Could you check a few things on this model? Use its own coordinates, in mm. A direction names the side the tool comes from. Round coordinates to 2 decimals unless told otherwise and drop trailing zeros. Order: outer loops, then holes, each group sorted by start corner. A loop starts at its lowest first (then second) coordinate and runs counter-clockwise, first axis right, second up. Notation, with made-up numbers: (34.25, -36.75) -> (41.25, -36.75) arc R24 ccw to (41.25, 1.25) -> close; hole circle Ø9 at (42, 8.25). An arc over 180 degrees is marked (long way). One line per question, with ' | ' between items.
```python
from build123d import *
from build123d.topology import SkipClean

# Parameters (mm, degrees)
SKETCH2_R           = 5.25
BOSS_EXTRUDE1_DEPTH = 14
CUT_EXTRUDE1_DEPTH  = 1
CUT_EXTRUDE2_DEPTH  = 1
BOSS_EXTRUDE2_DEPTH = 9
BOSS_EXTRUDE3_DEPTH = 9.5
FILLET1_R           = 1


with BuildPart() as part:
    # Sketch2 → Boss-Extrude1 (new body)
    with BuildSketch(Plane(origin=(0, 0, 0), x_dir=(0, 0, -1), z_dir=(1, 0, 0))):
        with BuildLine():
            ThreePointArc((0, 0), (9, 9), (0, 18))
            Line((0, 18), (-4.055355956, 18))
            Line((-4.055355956, 18), (-14.1, 8.3))
            Line((-14.1, 8.3), (-22.975773924, 5.754912782))
            ThreePointArc((-22.975773924, 5.754912782), (-23.743647767, 6.106105344), (-24.576075178, 6.24763647))
            Line((-24.576075178, 6.24763647), (-45.007968978, 23.392031022))
            Line((-45.007968978, 23.392031022), (-47.2, 21.2))
            Line((-47.2, 21.2), (-27.661634154, 1.661634154))
            ThreePointArc((-27.661634154, 1.661634154), (-25.892761453, -0.023213541), (-23.45, 0))
            Line((-23.45, 0), (0, 0))
        make_face()
        with Locations((0, 9)):
            Circle(SKETCH2_R, mode=Mode.SUBTRACT)
    extrude(amount=-BOSS_EXTRUDE1_DEPTH)

    # Sketch2_5 → Cut-Extrude1 (cut)
    with BuildSketch(Plane(origin=(0, 0, 0), x_dir=(0, 0, -1), z_dir=(1, 0, 0))):
        with BuildLine():
            Line((-29.259155366, 3.259155366), (-27.661634154, 1.661634154))
            ThreePointArc((-27.661634154, 1.661634154), (-27.396479719, 4.814248364), (-24.576075178, 6.24763647))
            Line((-24.576075178, 6.24763647), (-25.89413767, 7.35362222))
            ThreePointArc((-25.89413767, 7.35362222), (-25.722467199, 6.887608312), (-26.037233654, 6.503470587))
            ThreePointArc((-26.037233654, 6.503470587), (-27.626659815, 5.344602808), (-28.410825273, 3.540625374))
            ThreePointArc((-28.410825273, 3.540625374), (-28.748146118, 3.138148273), (-29.259155366, 3.259155366))
        make_face()
    extrude(amount=-CUT_EXTRUDE1_DEPTH, mode=Mode.SUBTRACT)

    # Sketch2_6 → Cut-Extrude2 (cut)
    with SkipClean():  # the faces are left unmerged after this step: merging them gives an invalid solid
        with BuildSketch(Plane(origin=(0, 0, 0), x_dir=(0, 0, -1), z_dir=(1, 0, 0))):
            with BuildLine():
                Line((-23.45, 0), (-21.263068229, 0))
                ThreePointArc((-21.263068229, 0), (-21.708634623, 0.273128697), (-21.667413143, 0.794117647))
                ThreePointArc((-21.667413143, 0.794117647), (-20.951415597, 3.103028999), (-21.793156226, 5.369126268))
                ThreePointArc((-21.793156226, 5.369126268), (-21.882671913, 5.8346109), (-21.543395734, 6.165640619))
                Line((-21.543395734, 6.165640619), (-22.975773924, 5.754912782))
                ThreePointArc((-22.975773924, 5.754912782), (-21.856917628, 4.574605546), (-21.45, 3))
                ThreePointArc((-21.45, 3), (-21.995836543, 1.197224362), (-23.45, 0))
            make_face()
        extrude(amount=-CUT_EXTRUDE2_DEPTH, mode=Mode.SUBTRACT)

    # Sketch3 → Boss-Extrude2 (add)
    with SkipClean():  # the faces are left unmerged after this step: merging them gives an invalid solid
        with BuildSketch(Plane.ZY.offset(14)):
            with BuildLine():
                ThreePointArc((23.45, 0), (21.46097847, 2.733092659), (22.975773924, 5.754912782))
                Line((22.975773924, 5.754912782), (14.1, 8.3))
                Line((14.1, 8.3), (11.259590113, 9.114474429))
                ThreePointArc((11.259590113, 9.114474429), (10.41329932, 8.974403731), (9.986911251, 8.230077781))
                ThreePointArc((9.986911251, 8.230077781), (9.041706899, 4.689696888), (6.886416056, 1.726180477))
                ThreePointArc((6.886416056, 1.726180477), (6.644893676, 0.629986809), (7.573920177, 0))
                Line((7.573920177, 0), (23.45, 0))
            make_face()
            with BuildLine():
                ThreePointArc((27.95, 3), (26.953857175, 5.341501193), (24.576075178, 6.24763647))
                ThreePointArc((24.576075178, 6.24763647), (23.743647767, 6.106105344), (22.975773924, 5.754912782))
                ThreePointArc((22.975773924, 5.754912782), (21.46097847, 2.733092659), (23.45, 0))
                ThreePointArc((23.45, 0), (25.892761453, -0.023213541), (27.661634154, 1.661634154))
                ThreePointArc((27.661634154, 1.661634154), (27.877090729, 2.315460374), (27.95, 3))
            make_face()
            with BuildLine():
                Line((47.2, 21.2), (45.007968978, 23.392031022))
                Line((45.007968978, 23.392031022), (24.576075178, 6.24763647))
                ThreePointArc((24.576075178, 6.24763647), (26.953857175, 5.341501193), (27.95, 3))
                ThreePointArc((27.95, 3), (27.877090729, 2.315460374), (27.661634154, 1.661634154))
                Line((27.661634154, 1.661634154), (47.2, 21.2))
            make_face()
        extrude(amount=BOSS_EXTRUDE2_DEPTH)

    # Sketch3_3 → Boss-Extrude3 (add)
    with SkipClean():  # the faces are left unmerged after this step: merging them gives an invalid solid
        with BuildSketch(Plane.ZY.offset(14)):
            with BuildLine():
                ThreePointArc((27.95, 3), (26.953857175, 5.341501193), (24.576075178, 6.24763647))
                ThreePointArc((24.576075178, 6.24763647), (23.743647767, 6.106105344), (22.975773924, 5.754912782))
                ThreePointArc((22.975773924, 5.754912782), (21.46097847, 2.733092659), (23.45, 0))
                ThreePointArc((23.45, 0), (25.892761453, -0.023213541), (27.661634154, 1.661634154))
                ThreePointArc((27.661634154, 1.661634154), (27.877090729, 2.315460374), (27.95, 3))
            make_face()
        extrude(amount=BOSS_EXTRUDE3_DEPTH)

    # Fillet1
    fillet1_edges = [part.edges().sort_by_distance(p)[0] for p in [
        (-7, 18, 4.055355956),
    ]]
    fillet(fillet1_edges, radius=FILLET1_R)


solid = part.part
```
1. I need wall thicknesses on probe 1 along X at (y, z) = (16, -0.5); probe 2 along Z at (x, y) = (-14.25, 2); probe 3 along Z at (x, y) = (-15, 18.25). Which ranges of each line are inside material? Lowest first, please.
From the geometry:
probe 1: x = -14 to 0 | probe 2: z = 7.16 to 28 | probe 3: z = 38.88 to 44.25
2. I want a section at A-A on z = -1. List the corners of the cut face in (x, y) for me.
From the geometry:
outline: (-14, 0.06) -> (0, 0.06) -> (0, 3.85) -> (-14, 3.85) -> close; (-14, 14.15) -> (0, 14.15) -> (0, 17.94) -> (-14, 17.94) -> close
3. I'm going to push flat-ended pins straight in: pin 1 (8 mm diameter, centred on x = -6.5, z = 16, fed in from +Y); pin 2 (2 mm diameter, centred on x = -8.5, z = 6, fed in from +Y); pin 3 (3 mm diameter, centred on x = -18, z = 35.5, fed in from -Y). Where does each tip first touch, or does it pass through?
From the geometry:
pin 1: stops at y = 10.33 | pin 2: stops at y = 17.09 | pin 3: stops at y = 8
4. I want a section at C-C on y = 16.5. List the corners of the cut face in (x, z) for me, and give its area (3 significant figures).
From the geometry:
outline: (-23, 36.79) -> (0, 36.79) -> (0, 42.5) -> (-23, 42.5) -> close; (-14, -4.97) -> (0, -4.97) -> (0, 5.61) -> (-14, 5.61) -> close | area: 279 mm²
5. On a 3-axis mill with a long thin cutter (end or side, diameter ignored), from which of +Z, -Z, +X, -X, +Y, -Y can I reach the whole of each face in a straight line? I mean faces 5 (the face through (-1, 3.1, 21.3)), 6 (the face through (-11, 0, 12)), 7 (the face through (-18.437, 0.646, 6.639)), 8 (the face through (-18.437, 4.736, 9.064)), 9 (the face through (-7, 18, 2)). Say none if no direction works.
From the geometry:
face 5: +X | face 6: -Z, +X, -X, -Y | face 7: -Z, -X | face 8: -Z, -X, +Y | face 9: -Z, +X, -X, +Y
6. I want a section at B-B on x = -6.25. List the corners of the cut face in (y, z) for me, and give its area (4 significant figures).
From the geometry:
outline: (0, 0) arc R9 ccw to (18, 0) -> (18, 3.65) arc R1 ccw to (17.72, 4.35) -> (8.3, 14.1) -> (5.75, 22.98) arc R3.25 ccw to (6.25, 24.58) -> (23.39, 45.01) -> (21.2, 47.2) -> (1.66, 27.66) arc R3.25 ccw to (0, 23.45) -> close; hole circle Ø10.5 at (9, 0) | area: 445.5 mm²
7. If we mould it in two halves opening along Z, with no side actions, what happens to faces 1 (the face through (-11.34, 14.7, 34.65)), 2 (the face through (-11, 12, 38)), 3 (the face through (-6.9, 13.08, 9.15)), 4 (the face through (0, 7, 7))? For each: pulls with the +Z half, pulls with the -Z half, needs draft (parallel to the pull), parting line crosses it, or undercut.
From the geometry:
face 1: undercut | face 2: pulls with the +Z half | face 3: undercut | face 4: needs draft
8. I want a section at D-D on y = 10.5. List the corners of the cut face in (x, z) for me, and give its area (3 significant figures).
From the geometry:
outline: (-23, 29.64) -> (0, 29.64) -> (0, 36.5) -> (-23, 36.5) -> close; (-14, -8.87) -> (0, -8.87) -> (0, -5.03) -> (-14, -5.03) -> close; (-14, 5.03) -> (0, 5.03) -> (0, 11.82) -> (-14, 11.82) -> close | area: 307 mm²
